Verification items for the finished model (mm, model axes). A direction names the side the tool comes from. Coordinates: 2 decimals unless noted, no trailing zeros. Order: outer loops, then holes, each group sorted by start corner. A loop starts at its lowest first (then second) coordinate and runs counter-clockwise, first axis right, second up. Notation, with made-up numbers: M 80.25,-34.75 L 134.25,-34.75 A18 ccw 134.25,-26.75 Z; hole C 71.25,-2.5 d3. An arc over 180 degrees is marked long. Answer as a JSON object with one key per item and string values. Group by question number.
(1) Material ranges on line 1 (Y direction, x = 10.5, z = 26); line 2 (Z direction, x = -58.5, y = 29); line 3 (X direction, y = 20.5, z = 86), recorded low to high.
(2) Mould release check, pull along Z, two halves, no side actions. Record for faces 1 (the face through (0, 23.5, 90)), 2 (the face through (0, 25, 100)), 3 (the face through (-1, -25, 5)): released by +Z, released by -Z, zero draft, split by the parting line, or undercut.
(3) Cross-section at B-B (z = 26.5). Enter the section's corners in (x, y).
(4) Gauge pin test, flat ends, axial feed: pin 1 Ø5 at (x, z) = (1, 88) entering from -Y; pin 2 Ø16.5 at (y, z) = (25, 36) entering from -X; pin 3 Ø1 at (x, y) = (25, 22) entering from +Z; pin 4 Ø6 at (y, z) = (12.5, 20) entering from -X. Record the tip position at first contact, or that the pin passes through.
(5) Access from +Z, -Z, +X, -X, +Y, -Y to the whole of each face (thin tool, end or side, straight path). Record for faces 4 (the face through (-75, 3, 5)), 5 (the face through (0, 17.5, 55)), 6 (the face through (-12.5, 25, 54)), 7 (the face through (12.5, 25, 54)).
(6) Cross-section at A-A (x = -30). Enter the section's corners in (y, z).
from build123d import *

# Parameters (mm, degrees)
SKETCH1_W           = 150
SKETCH1_H           = 50
BOSS_EXTRUDE1_DEPTH = 10
SKETCH2_W           = 25
SKETCH2_H           = 15
BOSS_EXTRUDE2_DEPTH = 90
SKETCH5_W           = 150
SKETCH5_H           = 10
BOSS_EXTRUDE3_DEPTH = 7.5


with BuildPart() as part:
    # Sketch1 → Boss-Extrude1 (new body)
    with BuildSketch(Plane.XY):
        Rectangle(SKETCH1_W, SKETCH1_H)
    extrude(amount=BOSS_EXTRUDE1_DEPTH)

    # Sketch2 → Boss-Extrude2 (add)
    with BuildSketch(Plane.XY.offset(10)):
        with Locations((0, 25)):
            Rectangle(SKETCH2_W, SKETCH2_H)
    extrude(amount=BOSS_EXTRUDE2_DEPTH)

    # Cut-Loft3: read off the stored shape, not the designer's step
    # Cut-Loft3: loft between two sections, ruled curve by curve
    cut_loft3_from = [
        Edge.make_bspline([(-3.437683222, 17.5, 85.082446333), (-13.272790555, 17.5, 91.957812777), (-6.397424111, 17.5, 101.792920111), (3.437683222, 17.5, 94.917553667), (13.272790555, 17.5, 88.042187223), (6.397424111, 17.5, 78.207079889), (-3.437683222, 17.5, 85.082446333)], [0, 0, 0, 0, 0.5, 0.5, 0.5, 1, 1, 1, 1], 3, [1, 0.333333333, 0.333333333, 1, 0.333333333, 0.333333333, 1]),
    ]
    cut_loft3_to = [
        Edge.make_bspline([(0, 23.5, 85), (-10, 23.5, 85), (-10, 23.5, 95), (0, 23.5, 95), (10, 23.5, 95), (10, 23.5, 85), (0, 23.5, 85)], [0, 0, 0, 0, 0.5, 0.5, 0.5, 1, 1, 1, 1], 3, [1, 0.333333333, 0.333333333, 1, 0.333333333, 0.333333333, 1]),
    ]
    cut_loft3 = Solid(Shell([*[Face.make_surface_from_curves(cut_loft3_from[k], cut_loft3_to[k]) for k in range(1)], Face(Wire(cut_loft3_from)), Face(Wire(cut_loft3_to))]))
    add(cut_loft3, mode=Mode.SUBTRACT)

    # Sketch5 → Boss-Extrude3 (add)
    with BuildSketch(Plane(origin=(0, 25, 0), x_dir=(1, 0, 0), z_dir=(0, 1, 0))):
        with Locations((0, -5)):
            Rectangle(SKETCH5_W, SKETCH5_H)
    extrude(amount=BOSS_EXTRUDE3_DEPTH)


solid = part.part
Taken from the geometry:
{
 "1": {"line 1": "y = 17.5 to 32.5", "line 2": "z = 0 to 10", "line 3": "x = -12.5 to -3.4, 3.4 to 12.5"},
 "2": {"face 1": "undercut", "face 2": "released by +Z", "face 3": "zero draft"},
 "3": {"outline": "M -12.5,17.5 L 12.5,17.5 L 12.5,32.5 L -12.5,32.5 Z"},
 "4": {"pin 1": "stops at y = 23.5", "pin 2": "stops at x = -12.5", "pin 3": "stops at z = 10", "pin 4": "passes through"},
 "5": {"face 4": "+Z, -Z, -X, +Y, -Y", "face 5": "+Z, +X, -X, -Y", "face 6": "+Z, -X, +Y, -Y", "face 7": "+Z, +X, +Y, -Y"},
 "6": {"outline": "M -25,0 L 32.5,0 L 32.5,10 L -25,10 Z"}
}
